The model under review builds one solid part; all positions refer to its coordinate system, in mm. A direction names the side the tool comes from. Coordinates: 2 decimals unless noted, no trailing zeros. Write each loop counter-clockwise with the first axis right and the second up, starting at its lowest first coordinate (ties: lowest second). Pieces come first, ordered by that corner, then holes. Notation, with made-up numbers: (-22.5, 1) - (-14.5, 1) arc R31 cw to (-14.5, 39) - close; hole circle Ø9 at (-14, -26.75). An arc over 180 degrees is marked (long way). Answer as CSV lines item,"result". Start each with the question number.
```python
from build123d import *

# Parameters (mm, degrees)
F1_DEPTH = 12
F2_R     = 3
F3_DEPTH = 20
F4_R     = 3
F5_DEPTH = 20
F6_W     = 30
F6_H     = 87
F7_DEPTH = 25


with BuildPart() as f1:
    # F0 (on Right) → F1 (new body)
    with BuildSketch(Plane.YZ):
        Polygon((0, 87), (0, 0), (60, 0), (100, 43.5), (60, 87), align=None)
    extrude(amount=F1_DEPTH)

    # F2 (on face) → F3 (cut)
    with BuildSketch(Plane.XY.offset(87)):
        with Locations((6, 45)):
            Circle(F2_R)
        with Locations((6, 15)):
            Circle(F2_R)
        with Locations((6, -15)):
            Circle(F2_R)
    extrude(amount=-F3_DEPTH, mode=Mode.SUBTRACT)

    # F4 (on face) → F5 (cut)
    with BuildSketch(Plane(origin=(0, 0, 0), x_dir=(1, 0, 0), z_dir=(0, 0, -1))):
        with BuildLine():
            ThreePointArc((9, -15), (8.12132, -12.87868), (6, -12))
            Line((6, -12), (6, -15))
            Line((6, -15), (6, -18))
            ThreePointArc((6, -18), (8.12132, -17.12132), (9, -15))
        make_face()
        with BuildLine():
            ThreePointArc((9, -45), (8.12132, -42.87868), (6, -42))
            Line((6, -42), (6, -45))
            Line((6, -45), (9, -45))
        make_face()
        with BuildLine():
            Line((6, -45), (6, -42))
            ThreePointArc((6, -42), (3, -45), (6, -48))
            Line((6, -48), (6, -45))
        make_face()
        with BuildLine():
            Line((6, -15), (6, -12))
            ThreePointArc((6, -12), (3, -15), (6, -18))
            Line((6, -18), (6, -15))
        make_face()
        with BuildLine():
            Line((9, -45), (6, -45))
            Line((6, -45), (6, -48))
            ThreePointArc((6, -48), (8.12132, -47.12132), (9, -45))
        make_face()
        with Locations((6, 15)):
            Circle(F4_R)
    extrude(amount=-F5_DEPTH, mode=Mode.SUBTRACT)

    # F6 (on face) → F7 (cut)
    with BuildSketch(Plane.YZ.offset(12)):
        with Locations((15, 43.5)):
            Rectangle(F6_W, F6_H)
    extrude(amount=-F7_DEPTH, mode=Mode.SUBTRACT)


solid = f1.part
```
(1) For pin 1 (5.5 mm diameter, centred on x = 6, y = 45, fed in from +Z); pin 2 (3 mm diameter, centred on x = 5, z = 23.5, fed in from +Y), all flat-tipped, find the tip position at first contact; note any pin that passes through.
(2) Add section C-C on x = 5. Give the boundary of the cut face in (y, z).
(3) The part is to be moulded in two halves that separate along X. For faces 1 (the cylindrical face through (6, 48, 77)), 2 (the flat face through (6, 30, 43)), 3 (the flat face through (0, 57, 44)), say which applies: released by +X, released by -X, zero draft, split by the parting line, or undercut.
(4) Add section D-D on y = 79. Give the boundary of the cut face in (x, z).
(5) Wall thickness on line 1 (Y direction, x = 6, z = 82); line 2 (Z direction, x = 7.25, y = 44.5); line 3 (X direction, y = 42.5, z = 68.5): over which ranges is each line inside the solid? List them lowest first.
(6) Add section A-A on x = 10.5. Give the boundary of the cut face in (y, z), then the cut area to 3 significant figures.
(7) For faces 4 (the flat face through (6, 45, 20)), 5 (the flat face through (6, 49, 87)), 6 (the flat face through (6, 45, 67)), list the 3-axis set-ups (+Z, -Z, +X, -X, +Y, -Y) from which the entire face can be reached by the end or side of a thin tool; tool diameter is ignored.
(8) Add section B-B on y = 46. Give the boundary of the cut face in (x, z).
Reported:
1,pin 1,"z = 67"
1,pin 2,"y = 82.99"
2,outline,"(30, 0) - (42.17, 0) - (42.17, 20) - (47.83, 20) - (47.83, 0) - (60, 0) - (100, 43.5) - (60, 87) - (47.83, 87) - (47.83, 67) - (42.17, 67) - (42.17, 87) - (30, 87) - close"
3,face 1,"undercut"
3,face 2,"zero draft"
3,face 3,"released by -X"
4,outline,"(0, 20.66) - (12, 20.66) - (12, 66.34) - (0, 66.34) - close"
5,line 1,"30 to 42, 48 to 64.6"
5,line 2,"20 to 67"
5,line 3,"0 to 4.34, 7.66 to 12"
6,outline,"(30, 0) - (60, 0) - (100, 43.5) - (60, 87) - (30, 87) - close"
6,area,"4,350 mm²"
7,face 4,"-Z"
7,face 5,"+Z, +X, -X, +Y, -Y"
7,face 6,"+Z"
8,outline,"(0, 0) - (3.17, 0) - (3.17, 20) - (8.83, 20) - (8.83, 0) - (12, 0) - (12, 87) - (8.83, 87) - (8.83, 67) - (3.17, 67) - (3.17, 87) - (0, 87) - close"
